```python
from build123d import *

# Parameters (mm, degrees)
ESBO_O1_R                = 14
ESBO_O1_R_2              = 1.25
RESSALTO_EXTRUS_O1_DEPTH = 3
ESBO_O4_R                = 10.5
RESSALTO_EXTRUS_O3_DEPTH = 50


with BuildPart() as part:
    # Esboço1 → Ressalto-extrusão1 (new body)
    with BuildSketch(Plane(origin=(0, 0, 0), x_dir=(1, 0, 0), z_dir=(0, 1, 0))):
        with Locations(Location((0, 0, 0), (0, 0, 270))):
            Circle(ESBO_O1_R)
        with Locations(Location((0, 11, 0), (0, 0, 270))):
            Circle(ESBO_O1_R_2, mode=Mode.SUBTRACT)
        with Locations(Location((7.778174593, 7.778174593, 0), (0, 0, 270))):
            Circle(ESBO_O1_R_2, mode=Mode.SUBTRACT)
        with Locations(Location((11, 0, 0), (0, 0, 270))):
            Circle(ESBO_O1_R_2, mode=Mode.SUBTRACT)
        with Locations(Location((7.778174593, -7.778174593, 0), (0, 0, 270))):
            Circle(ESBO_O1_R_2, mode=Mode.SUBTRACT)
        with Locations(Location((0, -11, 0), (0, 0, 270))):
            Circle(ESBO_O1_R_2, mode=Mode.SUBTRACT)
        with Locations(Location((-7.778174593, -7.778174593, 0), (0, 0, 270))):
            Circle(ESBO_O1_R_2, mode=Mode.SUBTRACT)
        with Locations(Location((-11, 0, 0), (0, 0, 270))):
            Circle(ESBO_O1_R_2, mode=Mode.SUBTRACT)
        with Locations(Location((-7.778174593, 7.778174593, 0), (0, 0, 270))):
            Circle(ESBO_O1_R_2, mode=Mode.SUBTRACT)
    extrude(amount=RESSALTO_EXTRUS_O1_DEPTH)

    # Loft1: read off the stored shape, not the designer's step
    # Loft1: loft between two sections, ruled curve by curve
    loft1_from = [
        Edge.make_bspline([(-7.155862372, 3, 2.245803579), (-2.664255213, 3, 16.557528323), (11.647469531, 3, 12.065921164), (7.155862372, 3, -2.245803579), (2.664255213, 3, -16.557528323), (-11.647469531, 3, -12.065921164), (-7.155862372, 3, 2.245803579)], [0, 0, 0, 0, 0.5, 0.5, 0.5, 1, 1, 1, 1], 3, [1, 0.333333333, 0.333333333, 1, 0.333333333, 0.333333333, 1]),
    ]
    loft1_to = [
        Edge.make_bspline([(-10.43066657, 33, -1.204655513), (-12.839977596, 33, 19.656677627), (8.021355544, 33, 22.065988653), (10.43066657, 33, 1.204655513), (12.839977596, 33, -19.656677627), (-8.021355544, 33, -22.065988653), (-10.43066657, 33, -1.204655513)], [0, 0, 0, 0, 0.5, 0.5, 0.5, 1, 1, 1, 1], 3, [1, 0.333333333, 0.333333333, 1, 0.333333333, 0.333333333, 1]),
    ]
    loft1 = Solid(Shell([*[Face.make_surface_from_curves(loft1_from[k], loft1_to[k]) for k in range(1)], Face(Wire(loft1_from)), Face(Wire(loft1_to))]))
    add(loft1)

    # Esboço4 → Ressalto-extrusão3 (add)
    with BuildSketch(Plane(origin=(0, 33, 0), x_dir=(1, 0, 0), z_dir=(0, 1, 0))):
        with Locations(Location((0, 0, 0), (0, 0, 173.412))):
            Circle(ESBO_O4_R)
    extrude(amount=RESSALTO_EXTRUS_O3_DEPTH)


solid = part.part
```
Build history of the part. All positions in model axes, mm. A direction names the side the tool comes from. Round coordinates to 2 decimals unless told otherwise and drop trailing zeros. Put each result on its own line as item: value.
Item 1: Wall check: probe 1 along X at (y, z) = (1.2, 0); probe 2 along Z at (x, y) = (0.5, 53); probe 3 along Y at (x, z) = (-9.5, -10.25). Give the ranges that are in metal, low to high. Write a range as from..to.
Here are the results:
probe 1: x = -14..-12.25, -9.75..9.75, 12.25..14
probe 2: z = -10.49..10.49
probe 3: y = 0..3
Item 2: Slice it at A-A, the plane x = 0. Count the separate pieces of the cut face and the enclosed holes in it, plus the area to 3 significant figures.
Here are the results:
separate pieces: 3
enclosed holes: 0
area: 1,650 mm^2
Item 3: Tool access for faces 4 (the face through (0, 83, 0)), 5 (the face through (12.24, 1.48, -0.16)), 6 (the face through (-9.174, 57.65, -5.108)): list every direction of +Z, -Z, +X, -X, +Y, -Y with a clear straight run to the whole face (end or side of a thin tool).
Here are the results:
face 4: +Z, -Z, +X, -X, +Y
face 5: -Y
face 6: +Y
Item 4: Flat gauge pins, fed straight in: P1, Ø1.5, axis at x = 7.5, z = -11, coming from the +Y side; P2, Ø8, axis at y = 12, z = -11, coming from the -X side; P3, Ø6, axis at y = 45.5, z = 10.5, coming from the -X side. Where does each tip first touch, or does it go through?
Here are the results:
P1: stops at y = 3
P2: stops at x = -4.36
P3: stops at x = -7.35
Item 5: Two-plate mould, pull along Z, no slides. Class faces 1 (the face through (0, 3, -8)), 2 (the face through (0.05, 1.48, 9.75)), 3 (the face through (-13.67, 1.48, -3.03)): pulls with the +Z half, pulls with the -Z half, needs draft (parallel to the pull), parting line crosses it, or undercut.
Here are the results:
face 1: needs draft
face 2: undercut
face 3: parting line crosses it
